Can you work these out from the drawing? Everything is in mm from the part's minimum corner. A direction names the side the tool comes from. Give positions to 0.01 mm unless a question says otherwise; leave off trailing zeros. Order: outer loops, then holes, each group sorted by start corner. A loop starts at its lowest first (then second) coordinate and runs counter-clockwise, first axis right, second up. Notation, with made-up numbers: (-27.75, -18) - (-15.75, -18) arc R33 cw to (-15.75, 12) - close; hole circle Ø1 at (35.25, -32.75). An arc over 180 degrees is marked (long way). Answer as a JSON object with one key per item and string values.
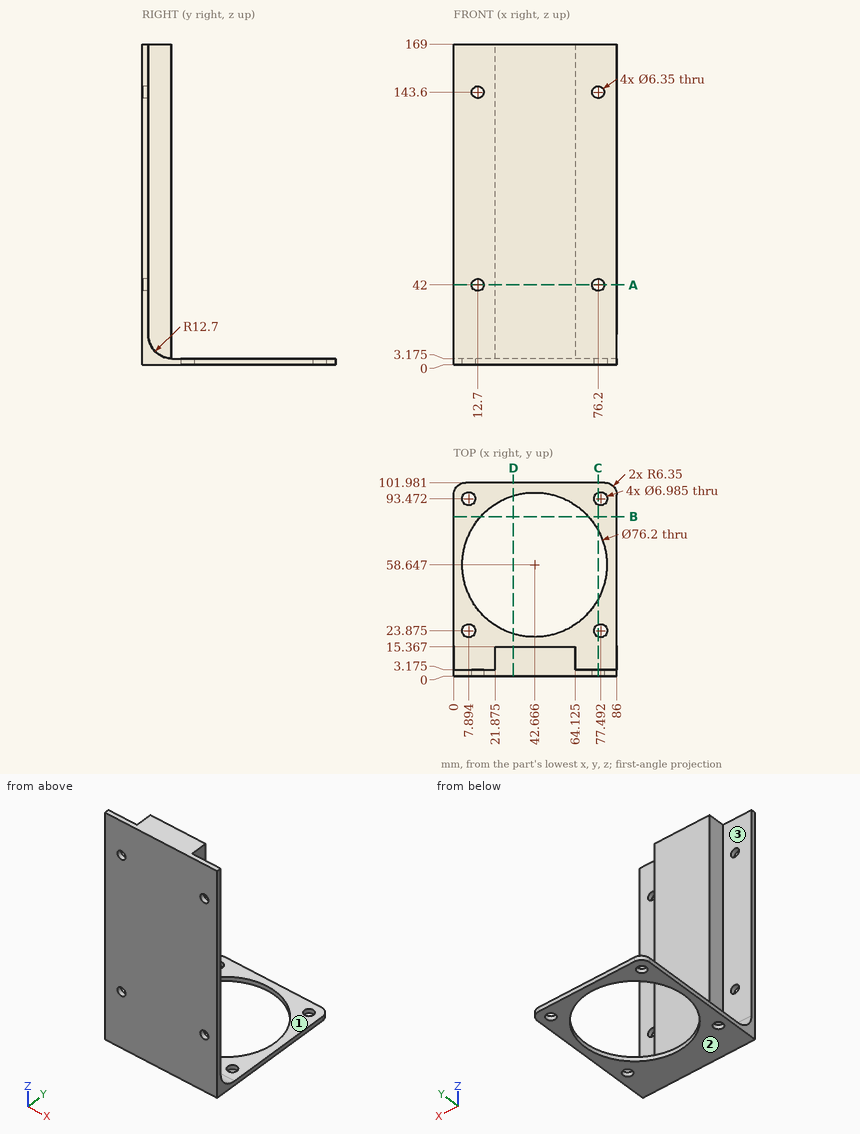
Q1. I'm going to push flat-ended pins straight in: pin 1 Ø10 at (x, z) = (76.2, 42) entering from +Y (1 decimal); pin 2 Ø6.5 at (x, y) = (77.49, 23.88) entering from -Z; pin 3 Ø8 at (x, z) = (57.5, 132.5) entering from +Y; pin 4 Ø2 at (y, z) = (14.5, 144.5) entering from -X (1 decimal). Where does each tip first touch, or does it pass through?
Recorded:
{"pin 1": "stops at y = 3.2", "pin 2": "passes through", "pin 3": "stops at y = 15.37", "pin 4": "stops at x = 21.9"}
Q2. If we section it at B-B, the plane y = 84: Please give me the cut outline in (x, z) (1 decimal).
Recorded:
{"outline": "(0, 0) - (14.2, 0) - (14.2, 3.2) - (0, 3.2) - close; (71.1, 0) - (86, 0) - (86, 3.2) - (71.1, 3.2) - close"}
Q3. If we section it at D-D, the plane x = 31.5: Please give me the cut outline in (y, z) (1 decimal).
Recorded:
{"outline": "(0, 0) - (22.2, 0) - (22.2, 3.2) - (15.9, 3.2) arc R12.7 cw to (15.4, 3.2) - (15.4, 169) - (0, 169) - close; (95.1, 0) - (102, 0) - (102, 3.2) - (95.1, 3.2) - close"}
Q4. If we section it at A-A, the plane z = 42: Please give me the cut outline in (x, y) (1 decimal).
Recorded:
{"outline": "(0, 0) - (9.5, 0) - (9.5, 3.2) - (0, 3.2) - close; (15.9, 0) - (73, 0) - (73, 3.2) - (64.1, 3.2) - (64.1, 15.4) - (21.9, 15.4) - (21.9, 3.2) - (15.9, 3.2) - close; (79.4, 0) - (86, 0) - (86, 3.2) - (79.4, 3.2) - close"}
Q5. I need wall thicknesses on L1, parallel to Z at x = 12.7, y = 1.45 (1 decimal); L2, parallel to X at y = 1, z = 143; L3, parallel to Y at x = 26, z = 127.5. Which ranges of each line are inside material? Lowest first, please.
Recorded:
{"L1": "z = 0 to 38.8, 45.2 to 140.4, 146.8 to 169", "L2": "x = 0 to 9.58, 15.82 to 73.08, 79.32 to 86", "L3": "y = 0 to 15.37"}
Q6. If we section it at C-C, the plane x = 76.2: Please give me the cut outline in (y, z) (1 decimal).
Recorded:
{"outline": "(0, 0) - (20.6, 0) - (20.6, 3.2) - (15.9, 3.2) arc R12.7 cw to (3.2, 15.9) - (3.2, 38.8) - (0, 38.8) - close; (0, 45.2) - (3.2, 45.2) - (3.2, 140.4) - (0, 140.4) - close; (0, 146.8) - (3.2, 146.8) - (3.2, 169) - (0, 169) - close; (27.1, 0) - (40.6, 0) - (40.6, 3.2) - (27.1, 3.2) - close; (76.7, 0) - (90.2, 0) - (90.2, 3.2) - (76.7, 3.2) - close; (96.7, 0) - (102, 0) - (102, 3.2) - (96.7, 3.2) - close"}
Q7. Which directions (+Z, -Z, +X, -X, +Y, -Y) give clear straight access to the entire face, cutting with the end or side of a thin tool? Please do the marked faces 1, 2 and 3.
Recorded:
{"face 1": "+Z, +X, -X, +Y", "face 2": "-Z, +X, -X, +Y, -Y", "face 3": "+Z, -X, +Y"}
